from build123d import *

# Parameters (mm, degrees)
BOSS_EXTRUDE1_DEPTH = 482.6
SHELL1_T            = -1.778


with BuildPart() as part:
    # Sketch1 → Boss-Extrude1 (new body)
    with BuildSketch(Plane.XY):
        with BuildLine():
            Line((0, 12.7), (0, 50.8))
            Line((0, 50.8), (16.51, 50.8))
            Line((16.51, 50.8), (16.51, 16.51))
            Line((16.51, 16.51), (50.8, 16.51))
            Line((50.8, 16.51), (50.8, 0))
            Line((50.8, 0), (12.7, 0))
            ThreePointArc((12.7, 0), (3.719743879, 3.719743879), (0, 12.7))
        make_face()
    extrude(amount=BOSS_EXTRUDE1_DEPTH)

    # Shell1
    shell1_openings = [part.faces().sort_by_distance(p)[0] for p in [
        (16.51, 33.655, 241.3),
        (33.655, 16.51, 241.3),
        (50.8, 8.255, 241.3),
        (8.255, 50.8, 241.3),
    ]]
    offset(amount=SHELL1_T, openings=shell1_openings, kind=Kind.INTERSECTION)


solid = part.part
Can you work these out from the model? Positions are in its coordinate system, mm. A direction names the side the tool comes from. Give positions to 0.01 mm unless a question says otherwise; leave off trailing zeros. Loops run counter-clockwise (first coordinate to the right, second up) from the corner with the lowest first, then second, coordinate; pieces in that order, holes last. Notation, with made-up numbers: (37.25, 26.25) -> (56.25, 26.25) arc R6 ccw to (56.25, 33.25) -> close; hole circle Ø4 at (24, 2). An arc over 180 degrees is marked (long way). Write item = value, one per line.
1) I need wall thicknesses on L1, parallel to Z at x = 4.5, y = 6.5; L2, parallel to X at y = 41, z = 92.5. Which ranges of each line are inside material? Lowest first, please. Write a range as from..to.
Check result:
L1 = 0..1.78, 480.82..482.6
L2 = 0..1.78
2) Will these pins go through, and if not, where does the flat tip stop? pin 1 (2 mm diameter, centred on x = 11, z = 111, fed in from +Y); pin 2 (12 mm diameter, centred on y = 36.5, z = 328, fed in from +X); pin 3 (1.4 mm diameter, centred on x = 42, z = 1, fed in from +Y).
Check result:
pin_1 = 2.12
pin_2 = 1.78
pin_3 = 16.51
3) Suppose I cut it at B-B on z = 368.5. Write out the boundary of the cut face in (x, y), then the cut area to 3 significant figures.
Check result:
outline = (0, 12.7) arc R12.7 ccw to (12.7, 0) -> (50.8, 0) -> (50.8, 1.78) -> (12.7, 1.78) arc R10.92 cw to (1.78, 12.7) -> (1.78, 50.8) -> (0, 50.8) -> close
area = 168 mm2
4) Suppose I cut it at A-A on y = 25.5. Write out the boundary of the cut face in (x, z).
Check result:
outline = (0, 0) -> (16.51, 0) -> (16.51, 1.78) -> (1.78, 1.78) -> (1.78, 480.82) -> (16.51, 480.82) -> (16.51, 482.6) -> (0, 482.6) -> close
5) For faces 1 (the flat face through (16, 21, 1.778)), 2 (the flat face through (50.8, 1, 240)), which set-ups out of +Z, -Z, +X, -X, +Y, -Y let a thin tool reach every point of the face, with its end or its side?
Check result:
face_1 = +X, +Y
face_2 = +Z, -Z, +X, +Y, -Y
